Can you work these out from the model? Positions are in its coordinate system, mm. Face numbers are marked on the shaded views. A direction names the side the tool comes from. Coordinates: 2 decimals unless noted, no trailing zeros. Loops run counter-clockwise (first coordinate to the right, second up) from the corner with the lowest first, then second, coordinate; pieces in that order, holes last.
```python
from build123d import *

# Parameters (mm, degrees)
SKETCH1_R           = 3
BOSS_EXTRUDE1_DEPTH = 10
SKETCH2_R           = 3
BOSS_EXTRUDE2_DEPTH = 2
BOSS_EXTRUDE3_DEPTH = 3


with BuildPart() as part:
    # Sketch1 → Boss-Extrude1 (new body)
    with BuildSketch(Plane.XY):
        Circle(SKETCH1_R)
        with BuildLine():
            Line((-1.161895004, 1.1), (1.161895004, 1.1))
            ThreePointArc((1.161895004, 1.1), (0, -1.6), (-1.161895004, 1.1))
        make_face(mode=Mode.SUBTRACT)
    extrude(amount=BOSS_EXTRUDE1_DEPTH)

    # Sketch2 → Boss-Extrude2 (add)
    with BuildSketch(Plane.XY.offset(10)):
        Circle(SKETCH2_R)
    extrude(amount=BOSS_EXTRUDE2_DEPTH)

    # Sketch3 → Boss-Extrude3 (add)
    with BuildSketch(Plane.XY.offset(12)):
        with BuildLine():
            Line((-1.702938637, 0.95), (1.702938637, 0.95))
            ThreePointArc((1.702938637, 0.95), (0, -1.95), (-1.702938637, 0.95))
        make_face()
    extrude(amount=BOSS_EXTRUDE3_DEPTH)


solid = part.part
```
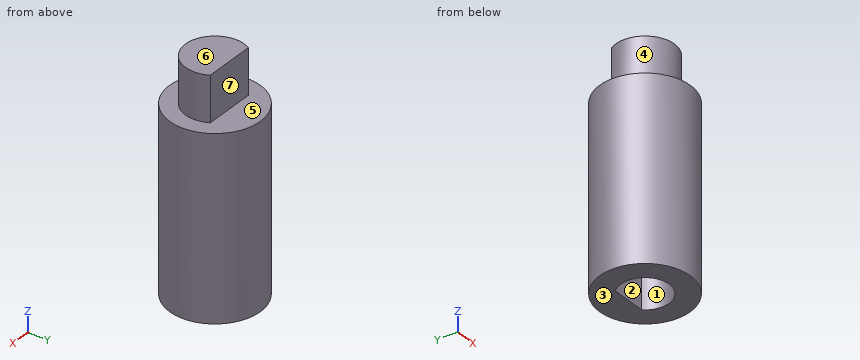
(1) If we mould it in two halves opening along X, with no side actions, what happens to the marked faces 1, 2, 3 and 4? For each: released by +X, released by -X, zero draft, split by the parting line, or undercut.
Check values:
face 1: undercut
face 2: undercut
face 3: zero draft
face 4: split by the parting line
(2) I want a section at B-B on y = 0. Write out the boundary of the cut face in (x, z).
Check values:
outline: (-3, 0) - (-1.6, 0) - (-1.6, 10) - (1.6, 10) - (1.6, 0) - (3, 0) - (3, 12) - (1.95, 12) - (1.95, 15) - (-1.95, 15) - (-1.95, 12) - (-3, 12) - close
(3) I want a section at D-D on x = -2.2. Write out the boundary of the cut face in (y, z).
Check values:
outline: (-2.04, 0) - (2.04, 0) - (2.04, 12) - (-2.04, 12) - close
(4) If I drill on probe 1 along Z at (x, y) = (1.15, 0.4); probe 2 along Z at (x, y) = (2.1, 1.25); probe 3 along Y at (x, z) = (1.3, 4.5), over which ranges is the centre line in solid material (lowest first)?
Check values:
probe 1: z = 10 to 15
probe 2: z = 0 to 12
probe 3: y = -2.7 to -0.93, 0.93 to 2.7
(5) I'm going to push flat-ended pins straight in: pin 1 (2 mm diameter, centred on y = 2, z = 11, fed in from +X); pin 2 (2 mm diameter, centred on x = 0, y = 0, fed in from -Z); pin 3 (1.5 mm diameter, centred on x = -0.5, z = 13, fed in from +Y). Where does each tip first touch, or does it pass through?
Check values:
pin 1: stops at x = 2.83
pin 2: stops at z = 10
pin 3: stops at y = 0.95
(6) Which directions (+Z, -Z, +X, -X, +Y, -Y) give clear straight access to the entire face, cutting with the end or side of a thin tool? Please do the marked faces 5, 6 and 7.
Check values:
face 5: +Z
face 6: +Z, +X, -X, +Y, -Y
face 7: +Z, +X, -X, +Y
(7) I want a section at A-A on x = 0. Write out the boundary of the cut face in (y, z), then the cut area to 3 significant figures.
Check values:
outline: (-3, 0) - (-1.6, 0) - (-1.6, 10) - (1.1, 10) - (1.1, 0) - (3, 0) - (3, 12) - (0.95, 12) - (0.95, 15) - (-1.95, 15) - (-1.95, 12) - (-3, 12) - close
area: 53.7 mm2
(8) I want a section at C-C on y = -2.6. Write out the boundary of the cut face in (x, z), then the cut area to 3 significant figures.
Check values:
outline: (-1.5, 0) - (1.5, 0) - (1.5, 12) - (-1.5, 12) - close
area: 35.9 mm2
